Study the drawing (mm; zero at the part's minimum x, y, z) and answer. A direction names the side the tool comes from. Coordinates: 2 decimals unless noted, no trailing zeros. Write each loop counter-clockwise with the first axis right and the second up, starting at its lowest first coordinate (ties: lowest second). Pieces come first, ordered by that corner, then holes. Notation, with made-up numbers: (86, 59) -> (116, 59) arc R17 cw to (116, 81) -> close; hole circle Ø7 at (74, -2.5). An arc over 180 degrees is marked (long way). Write item = value, one per line. Start each with the question number.
1) A tool of negligible diameter and unlimited length cuts with its end or side. For the marked faces 1, 2, 3, 4 and 5, from which of +Z, -Z, +X, -X, +Y, -Y can it reach the whole face along a straight path? Write none if from no direction.
2) Section C-C (y = 32) is taken. Determine the outline of the cut face in (x, z), plus the area to 3 significant figures.
3) Section A-A (z = 13) is taken. Determine the outline of the cut face in (x, y), plus the area to 3 significant figures.
4) Find the intervals of material crossed by line 1 along Z through (x, y) = (17.5, 2.5); line 2 along Y through (x, z) = (31.5, 23.5); line 3 along X through (y, z) = (37, 35), in increasing order. Write a range as from..to.
5) For a pull along Y with two mould halves and no side action, classify the marked faces 6, 7 and 8 as released by +Y, released by -Y, zero draft, split by the parting line, or undercut.
6) Flat-ended cylindrical pins translate along their axes: pin 1 Ø10 at (x, z) = (42.5, 35) entering from -Y; pin 2 Ø10 at (y, z) = (33.5, 17.5) entering from +X; pin 3 Ø2 at (x, y) = (64, 29.5) entering from +Z; pin 4 Ø6 at (y, z) = (9.5, 46.5) entering from +X. Find the tip coordinate at first contact, or state that the pin passes through.
7) Section D-D (z = 6) is taken. Determine the outline of the cut face in (x, y).
8) Section B-B (x = 80.5) is taken. Determine the outline of the cut face in (y, z), plus the area to 3 significant figures.
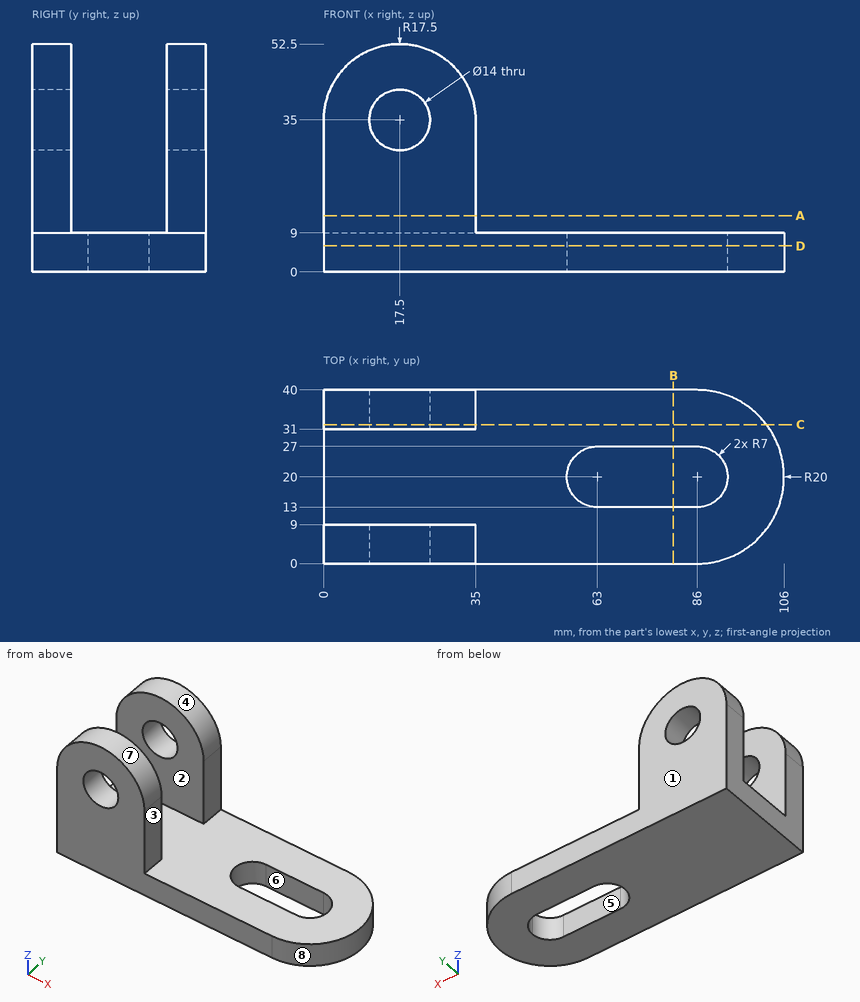
Answer key:
q1.face_1 = +Z, -Z, +X, -X, +Y
q1.face_2 = +Z, +X, -X
q1.face_3 = +Z, +X, +Y, -Y
q1.face_4 = +Z, +Y, -Y
q1.face_5 = +Z, -Z
q2.outline = (0, 0) -> (102, 0) -> (102, 9) -> (35, 9) -> (35, 35) arc R17.5 ccw to (0, 35) -> close; hole circle Ø14 at (17.5, 35)
q2.area = 2,160 mm^2
q3.outline = (0, 0) -> (35, 0) -> (35, 9) -> (0, 9) -> close; (0, 31) -> (35, 31) -> (35, 40) -> (0, 40) -> close
q3.area = 630 mm^2
q4.line_1 = 0..28, 42..52.5
q4.line_2 = 0..9, 31..40
q4.line_3 = 0..10.5, 24.5..35
q5.face_6 = undercut
q5.face_7 = zero draft
q5.face_8 = split by the parting line
q6.pin_1 = through
q6.pin_2 = 35
q6.pin_3 = 9
q6.pin_4 = 32.77
q7.outline = (0, 0) -> (86, 0) arc R20 ccw to (86, 40) -> (0, 40) -> close; hole (63, 13) -> (86, 13) arc R7 ccw to (86, 27) -> (63, 27) arc R7 ccw to start
q8.outline = (0, 0) -> (13, 0) -> (13, 9) -> (0, 9) -> close; (27, 0) -> (40, 0) -> (40, 9) -> (27, 9) -> close
q8.area = 234 mm^2
